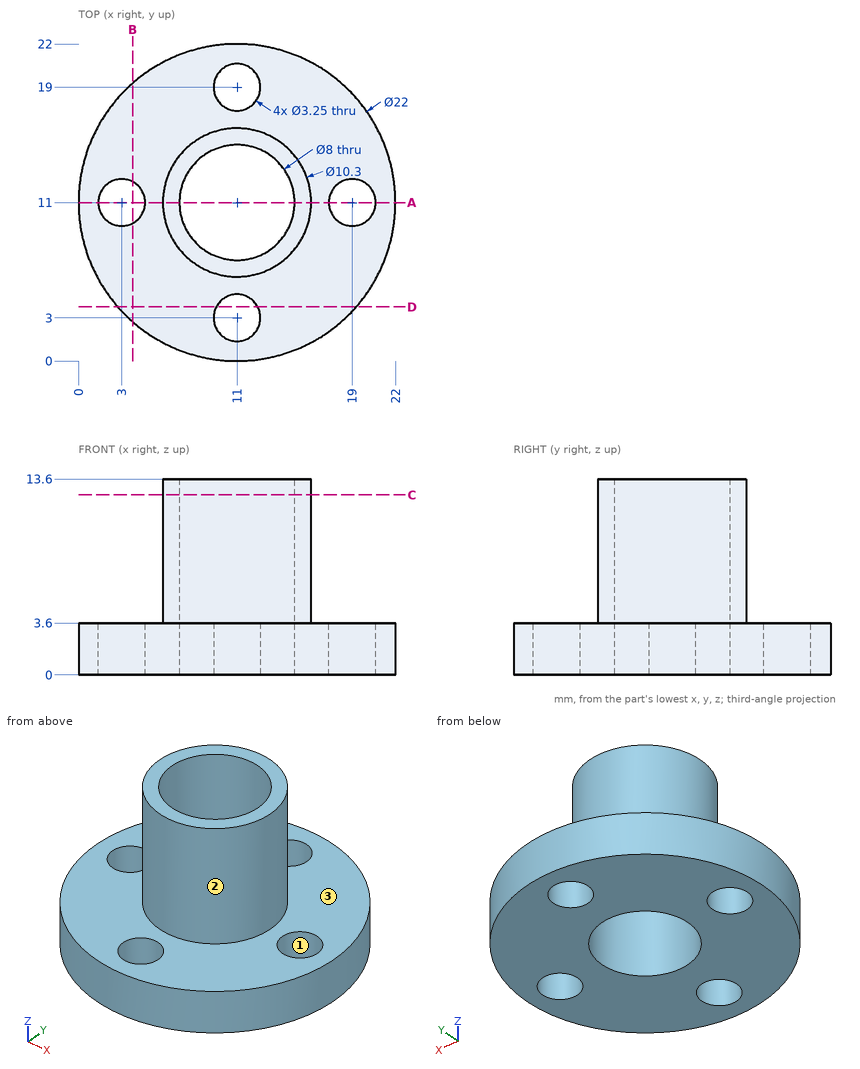
Print and shaded views of the part. All mm, measured from the part's lowest x, y and z. Give positions to 0.01 mm unless a question says otherwise; leave off trailing zeros. Loops run counter-clockwise (first coordinate to the right, second up) from the corner with the lowest first, then second, coordinate; pieces in that order, holes last. Notation, with made-up numbers: (15.5, -1) - (70.5, -1) arc R26 ccw to (70.5, 21) - close; hole circle Ø2 at (42, 14). An arc over 180 degrees is marked (long way). One line per item, written item: value. Start each with the question number.
1. Slice it at C-C (z = 12.5). List the corners of the cut face in (x, y).
2. Pull direction Y, two halves, no side cores. Call the marked faces 1, 2 and 3: pulls with the +Y half, pulls with the -Y half, needs draft (parallel to the pull), parting line crosses it, or undercut.
3. Slice it at A-A (y = 11). List the corners of the cut face in (x, z) (3 decimals).
4. Pin check, flat tips, straight feed: pin 1 (4 mm diameter, centred on y = 5, z = 3, fed in from +X); pin 2 (5 mm diameter, centred on x = 6, z = 10, fed in from -Y); pin 3 (1 mm diameter, centred on x = 9, z = 7, fed in from +Y). Stop position of each tip, or through.
5. Slice it at B-B (x = 3.75). List the corners of the cut face in (y, z), plus the area to 3 significant figures.
6. Probe L1, parallel to Y at x = 11, z = 2.15 (3 decimals); L2, parallel to Y at x = 11, z = 7.25; L3, parallel to Z at x = 14.25, y = 17.5. List the from-to ranges inside material, lowest first. Write a range as from..to.
Solution:
1. outline: circle Ø10.3 at (11, 11); hole circle Ø8 at (11, 11)
2. face 1: undercut
2. face 2: parting line crosses it
2. face 3: needs draft
3. outline: (0, 0) - (1.375, 0) - (1.375, 3.6) - (0, 3.6) - close; (4.625, 0) - (7, 0) - (7, 13.6) - (5.85, 13.6) - (5.85, 3.6) - (4.625, 3.6) - close; (15, 0) - (17.375, 0) - (17.375, 3.6) - (16.15, 3.6) - (16.15, 13.6) - (15, 13.6) - close; (20.625, 0) - (22, 0) - (22, 3.6) - (20.625, 3.6) - close
4. pin 1: stops at x = 21.25
4. pin 2: stops at y = 6.5
4. pin 3: stops at y = 15.93
5. outline: (2.73, 0) - (9.56, 0) - (9.56, 3.6) - (2.73, 3.6) - close; (12.44, 0) - (19.27, 0) - (19.27, 3.6) - (12.44, 3.6) - close
5. area: 49.2 mm^2
6. L1: y = 0..1.375, 4.625..7, 15..17.375, 20.625..22
6. L2: y = 5.85..7, 15..16.15
6. L3: z = 0..3.6
